Part model, mm, in its own coordinate system. A direction names the side the tool comes from. Give positions to 0.01 mm unless a question says otherwise; leave off trailing zeros. Order: outer loops, then holes, each group sorted by start corner. A loop starts at its lowest first (then second) coordinate and runs counter-clockwise, first axis right, second up. Notation, with made-up numbers: (56, 33) - (111, 33) arc R27 cw to (111, 53) - close; hole circle Ø9 at (-14.75, 81.5). An arc over 180 degrees is marked (long way). One line per item, written item: value.
```python
from build123d import *

# Parameters (mm, degrees)
F0_W     = 165.1
F0_H     = 88.9
F0_W_2   = 152.4
F0_H_2   = 76.2
F1_DEPTH = 76.2
F0_W_3   = 47.244
F0_H_3   = 34.29
F0_W_4   = 47.498
F2_DEPTH = 76.2
F3_R     = 10.16
F4_W     = 177.8
F4_H     = 101.6
F5_DEPTH = 12.7
F6_R     = 10.16


# Not quite as in the source:
# - a feature names something its author has since deleted; it is built from what else it names


with BuildPart() as f1:
    # F0 (on Front) → F1 (new body)
    with BuildSketch(Plane.XZ):
        Rectangle(F0_W, F0_H)
        Rectangle(F0_W_2, F0_H_2, mode=Mode.SUBTRACT)
    extrude(amount=F1_DEPTH)

    # F0 (on Front) → F2 (join)
    with BuildSketch(Plane.XZ):
        Rectangle(F0_W_2, F0_H_2)
        with Locations((-50.038, -18.415)):
            Rectangle(F0_W_3, F0_H_3, mode=Mode.SUBTRACT)
        with Locations((-0.127, -18.415)):
            Rectangle(F0_W_4, F0_H_3, mode=Mode.SUBTRACT)
        with Locations((49.911, -18.415)):
            Rectangle(F0_W_4, F0_H_3, mode=Mode.SUBTRACT)
        with Locations((-50.038, 18.415)):
            Rectangle(F0_W_3, F0_H_3, mode=Mode.SUBTRACT)
        with Locations((-0.127, 18.415)):
            Rectangle(F0_W_4, F0_H_3, mode=Mode.SUBTRACT)
        with Locations((49.911, 18.415)):
            Rectangle(F0_W_4, F0_H_3, mode=Mode.SUBTRACT)
    extrude(amount=F2_DEPTH)

    # F3
    f3_edges = [f1.edges().sort_by_distance(p)[0] for p in [
        (-82.55, -38.1, -44.45),
        (82.55, -38.1, -44.45),
        (-82.55, -38.1, 44.45),
        (82.55, -38.1, 44.45),
    ]]
    fillet(f3_edges, radius=F3_R)

    # F4 (on Front) → F5 (join)
    with BuildSketch(Plane.XZ):
        Rectangle(F4_W, F4_H)
    extrude(amount=F5_DEPTH)

    # F6
    f6_edges = [f1.edges().sort_by_distance(p)[0] for p in [
        (-88.9, -6.35, 50.8),
        (88.9, -6.35, 50.8),
        (-88.9, -6.35, -50.8),
        (88.9, -6.35, -50.8),
    ]]
    fillet(f6_edges, radius=F6_R)


solid = f1.part
```
1) Cut at B-B, the plane z = -27. Give the cut face in (x, y).
Outcome:
outline: (-88.9, -12.7) - (-82.55, -12.7) - (-82.55, -76.2) - (-73.66, -76.2) - (-73.66, -12.7) - (-26.42, -12.7) - (-26.42, -76.2) - (-23.88, -76.2) - (-23.88, -12.7) - (23.62, -12.7) - (23.62, -76.2) - (26.16, -76.2) - (26.16, -12.7) - (73.66, -12.7) - (73.66, -76.2) - (82.55, -76.2) - (82.55, -12.7) - (88.9, -12.7) - (88.9, 0) - (-88.9, 0) - close
2) Cut at A-A, the plane y = -68. Give the number of separate pieces and of enclosed holes in the cut face, then the cut area to 3 significant figures.
Outcome:
separate pieces: 1
enclosed holes: 6
area: 4,830 mm^2
3) Drill centre lines: line 1 along Z through (x, y) = (50, -45); line 2 along X through (y, z) = (-60, 14); line 3 along Y through (x, z) = (5, -19.5). Where is each one in solid material? Low to high. Write a range as from..to.
Outcome:
line 1: z = -44.45..-35.56, -1.27..1.27, 35.56..44.45
line 2: x = -82.55..-73.66, -26.42..-23.88, 23.62..26.16, 73.66..82.55
line 3: y = -12.7..0
4) Cut at C-C, the plane x = 8.5. Give the cut face in (y, z).
Outcome:
outline: (-76.2, -44.45) - (-12.7, -44.45) - (-12.7, -50.8) - (0, -50.8) - (0, 50.8) - (-12.7, 50.8) - (-12.7, 44.45) - (-76.2, 44.45) - (-76.2, 35.56) - (-12.7, 35.56) - (-12.7, 1.27) - (-76.2, 1.27) - (-76.2, -1.27) - (-12.7, -1.27) - (-12.7, -35.56) - (-76.2, -35.56) - close
5) Which spindle directions (+Z, -Z, +X, -X, +Y, -Y) get a long thin tool onto all of the face, cutting with end or side? Do faces 1 (the flat face through (0, -12.7, -18)), 2 (the cylindrical face through (79.495, -44.894, 41.553)), 3 (the flat face through (-1, -6, -50.8)), 4 (the cylindrical face through (79.495, -44.894, -41.553)), 5 (the cylindrical face through (85.845, -6.439, 47.903)). Say none if no direction does.
Outcome:
face 1: -Y
face 2: +Z, +X, -Y
face 3: -Z, +X, -X, +Y, -Y
face 4: -Z, +X, -Y
face 5: +Z, +X, +Y, -Y
6) Mould opens along X. For faces 6 (the flat face through (-50, -12.7, -18)), 7 (the flat face through (88.9, -6, -1)), 8 (the cylindrical face through (-86.003, -6.439, 47.745)) say: released by +X, released by -X, zero draft, split by the parting line, or undercut.
Outcome:
face 6: undercut
face 7: released by +X
face 8: released by -X
7) Pin check, flat tips, straight feed: pin 1 (4 mm diameter, centred on y = -34, z = -28, fed in from +X); pin 2 (1 mm diameter, centred on y = -58, z = -14.5, fed in from -X); pin 3 (1 mm diameter, centred on x = 13, z = -20, fed in from +Y); pin 4 (17 mm diameter, centred on x = -51, z = -26.5, fed in from -Y). Stop position of each tip, or through.
Outcome:
pin 1: stops at x = 82.55
pin 2: stops at x = -82.55
pin 3: stops at y = 0
pin 4: stops at y = -12.7
